The model under review builds one solid part; all positions refer to its coordinate system, in mm. Face numbers are marked on the shaded views. A direction names the side the tool comes from. Give positions to 0.01 mm unless a question says otherwise; leave off trailing zeros. Write each loop counter-clockwise with the first axis right and the second up, starting at its lowest first coordinate (ties: lowest second). Pieces come first, ordered by that corner, then holes. Notation, with made-up numbers: (40.25, 87) - (73.25, 87) arc R23 ccw to (73.25, 102) - close; hole circle Ø4 at (71.5, 68.25). An arc over 180 degrees is marked (long way). Write item = value, one per line.
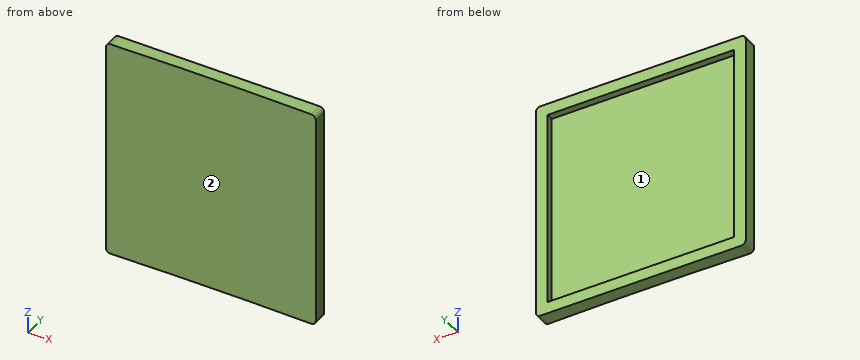
```python
from build123d import *

# Parameters (mm, degrees)
BOSS_EXTRUDE1_DEPTH     = 3
CUT_EXTRUDE1_DEPTH      = 33.672618505
CUT_EXTRUDE1_DEPTH_BACK = 33.672618505
SKETCH4_W               = 40
SKETCH4_H               = 42
CUT_EXTRUDE2_DEPTH      = 1.5


with BuildPart() as part:
    # Sketch1 → Boss-Extrude1 (new body)
    with BuildSketch(Plane(origin=(0, 0, 0), x_dir=(1, 0, 0), z_dir=(0, 1, 0))):
        with BuildLine():
            Line((21.5, 23.5), (-21.5, 23.5))
            ThreePointArc((-21.5, 23.5), (-22.207106781, 23.207106781), (-22.5, 22.5))
            Line((-22.5, 22.5), (-22.5, -22.5))
            ThreePointArc((-22.5, -22.5), (-22.207106781, -23.207106781), (-21.5, -23.5))
            Line((-21.5, -23.5), (21.5, -23.5))
            ThreePointArc((21.5, -23.5), (22.207106781, -23.207106781), (22.5, -22.5))
            Line((22.5, -22.5), (22.5, 22.5))
            ThreePointArc((22.5, 22.5), (22.207106781, 23.207106781), (21.5, 23.5))
        make_face()
    extrude(amount=-BOSS_EXTRUDE1_DEPTH)

    # Sketch2 → Cut-Extrude1 (cut, two sides: drawn at the far end of the back side and taken through both)
    with BuildSketch(Plane.XY.offset(-CUT_EXTRUDE1_DEPTH_BACK)):
        with BuildLine():
            Line((-22.5, -3), (22.5, -3))
            ThreePointArc((22.5, -3), (0, -2.75), (-22.5, -3))
        make_face()
    extrude(amount=CUT_EXTRUDE1_DEPTH + CUT_EXTRUDE1_DEPTH_BACK, mode=Mode.SUBTRACT)

    # Sketch4 → Cut-Extrude2 (cut)
    with BuildSketch(Plane(origin=(0, 0, 0), x_dir=(1, 0, 0), z_dir=(0, 1, 0))):
        Rectangle(SKETCH4_W, SKETCH4_H)
    extrude(amount=-CUT_EXTRUDE2_DEPTH, mode=Mode.SUBTRACT)


solid = part.part
```
1. Machinability: for the marked faces 1 and 2, which of the approach directions +Z, -Z, +X, -X, +Y, -Y give a long, thin tool a straight path to every point of the face, cutting with its end or side? Answer none if there is none.
Findings below:
face_1 = +Y
face_2 = +Z, -Z, -Y
2. For line 1 (X direction, y = -0.3, z = 18.5); line 2 (Z direction, x = 16, y = -0.75); line 3 (Y direction, x = 3, z = -20), list the stretches that pass through material, from the lowest coordinate up. Write a range as from..to.
Findings below:
line_1 = -22.5..-20, 20..22.5
line_2 = -23.5..-21, 21..23.5
line_3 = -2.75..-1.5
3. Take a section at B-B on z = 3. Give the boundary of the cut face in (x, y) (3 decimals).
Findings below:
outline = (-22.5, -3) arc R1012.625 cw to (22.5, -3) - (22.5, 0) - (20, 0) - (20, -1.5) - (-20, -1.5) - (-20, 0) - (-22.5, 0) - close
4. Insertion check: P1, Ø12, axis at x = 10.5, z = 4.5, coming from the -Y side; P2, Ø20, axis at x = -9, z = 7, coming from the +Y side. Each pin has a flat end and moves straight along its axis. Give the tip position at first contact, or say it passes through.
Findings below:
P1 = -2.88
P2 = -1.5
5. Take a section at A-A on x = -18. Give the boundary of the cut face in (y, z).
Findings below:
outline = (-2.91, -23.5) - (0, -23.5) - (0, -21) - (-1.5, -21) - (-1.5, 21) - (0, 21) - (0, 23.5) - (-2.91, 23.5) - close
